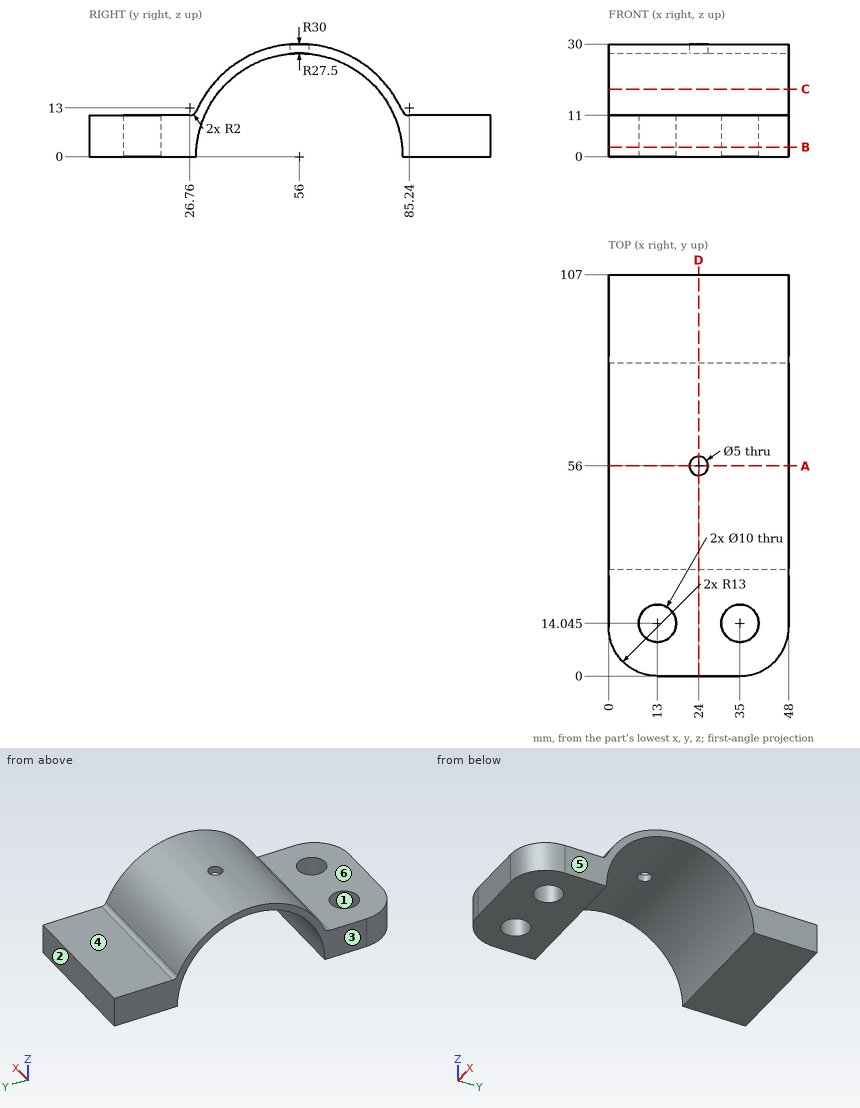
Could you check a few things on this drawing? It's one solid part, dimensions in mm from its lowest x, y, z. A direction names the side the tool comes from. Round coordinates to 2 decimals unless told otherwise and drop trailing zeros. Write each loop counter-clockwise with the first axis right and the second up, starting at its lowest first coordinate (ties: lowest second). Pieces come first, ordered by that corner, then holes. Notation, with made-up numbers: (57.5, 58.5) -> (64.5, 58.5) arc R18 cw to (64.5, 78.5) -> close; hole circle Ø3 at (22.5, 15). An arc over 180 degrees is marked (long way). One line per item, written item: value.
1) For the marked faces 4, 5 and 6, which set-ups out of +Z, -Z, +X, -X, +Y, -Y let a thin tool reach every point of the face, with its end or its side?
Filled sheet:
face 4: +Z, +X, -X, +Y
face 5: +Z, -Z, +X, +Y, -Y
face 6: +Z, +X, -X, -Y
2) We'd pull the mould along X, two halves only. Please class the marked faces 1, 2 and 3: released by +X, released by -X, zero draft, split by the parting line, or undercut.
Filled sheet:
face 1: undercut
face 2: zero draft
face 3: released by -X
3) Suppose I cut it at B-B on z = 2.5. List the corners of the cut face in (x, y) for me (1 decimal).
Filled sheet:
outline: (0, 13) arc R13 ccw to (13, 0) -> (35, 0) arc R13 ccw to (48, 13) -> (48, 28.6) -> (0, 28.6) -> close; (0, 83.4) -> (48, 83.4) -> (48, 107) -> (0, 107) -> close; hole circle Ø10 at (13, 14); hole circle Ø10 at (35, 14)
4) Suppose I cut it at C-C on z = 18. List the corners of the cut face in (x, y) for me.
Filled sheet:
outline: (0, 32) -> (48, 32) -> (48, 35.21) -> (0, 35.21) -> close; (0, 76.79) -> (48, 76.79) -> (48, 80) -> (0, 80) -> close
5) Suppose I cut it at A-A on y = 56. List the corners of the cut face in (x, z) for me.
Filled sheet:
outline: (0, 27.5) -> (21.5, 27.5) -> (21.5, 30) -> (0, 30) -> close; (26.5, 27.5) -> (48, 27.5) -> (48, 30) -> (26.5, 30) -> close
6) If I drill on line 1 (Z direction, x = 43, y = 97); line 2 (Y direction, x = 44.5, z = 2.5) (1 decimal); line 3 (Y direction, x = 11, z = 23) (1 decimal), over which ranges is the centre line in solid material (lowest first)? Write a range as [from, to].
Filled sheet:
line 1: z = [0, 11]
line 2: y = [4.1, 28.6], [83.4, 107]
line 3: y = [36.7, 40.9], [71.1, 75.3]
7) Suppose I cut it at D-D on x = 24. List the corners of the cut face in (y, z) for me (1 decimal).
Filled sheet:
outline: (0, 0) -> (28.5, 0) arc R27.5 cw to (53.5, 27.4) -> (53.5, 29.9) arc R30 ccw to (28.6, 12.2) arc R2 cw to (26.8, 11) -> (0, 11) -> close; (58.5, 27.4) arc R27.5 cw to (83.5, 0) -> (107, 0) -> (107, 11) -> (85.2, 11) arc R2 cw to (83.4, 12.2) arc R30 ccw to (58.5, 29.9) -> close
8) I'm going to push flat-ended pins straight in: pin 1 Ø16 at (x, y) = (35, 14.04) entering from +Z; pin 2 Ø8 at (x, y) = (21, 43.5) entering from -Z; pin 3 Ø12 at (x, z) = (42.5, 26.5) entering from +Y; pin 4 Ø11.5 at (x, y) = (13, 14.04) entering from -Z. Where does each tip first touch, or does it pass through?
Filled sheet:
pin 1: stops at z = 11
pin 2: stops at z = 22
pin 3: stops at y = 77.9
pin 4: stops at z = 0
